Check sheet for the drawn part. Datum: minimum x, y, z corner. Units: mm. Round coordinates to 2 decimals unless told otherwise and drop trailing zeros. Write each loop counter-clockwise with the first axis right and the second up, starting at its lowest first coordinate (ties: lowest second). Pieces come first, ordered by that corner, then holes. Notation, with made-up numbers: M 65,35.5 L 83,35.5 A9 cw 83,48.5 Z; hole C -8,-4 d4. An arc over 180 degrees is marked long. One line per item, written item: value. Start each with the question number.
Item 1: Section check C-C, the plane y = 112. Record the cut outline in (x, z), then the cut area to 3 significant figures.
Item 2: Section check B-B, the plane z = 189. Record the cut outline in (x, y), then the cut area to 3 significant figures.
Item 3: Thickness scan on probe 1 along Z at (x, y) = (5.75, 103.5); probe 2 along Y at (x, z) = (1.5, 250); probe 3 along Y at (x, z) = (5.75, 187). Record the ranges inside material, lowest first. Write a range as from..to.
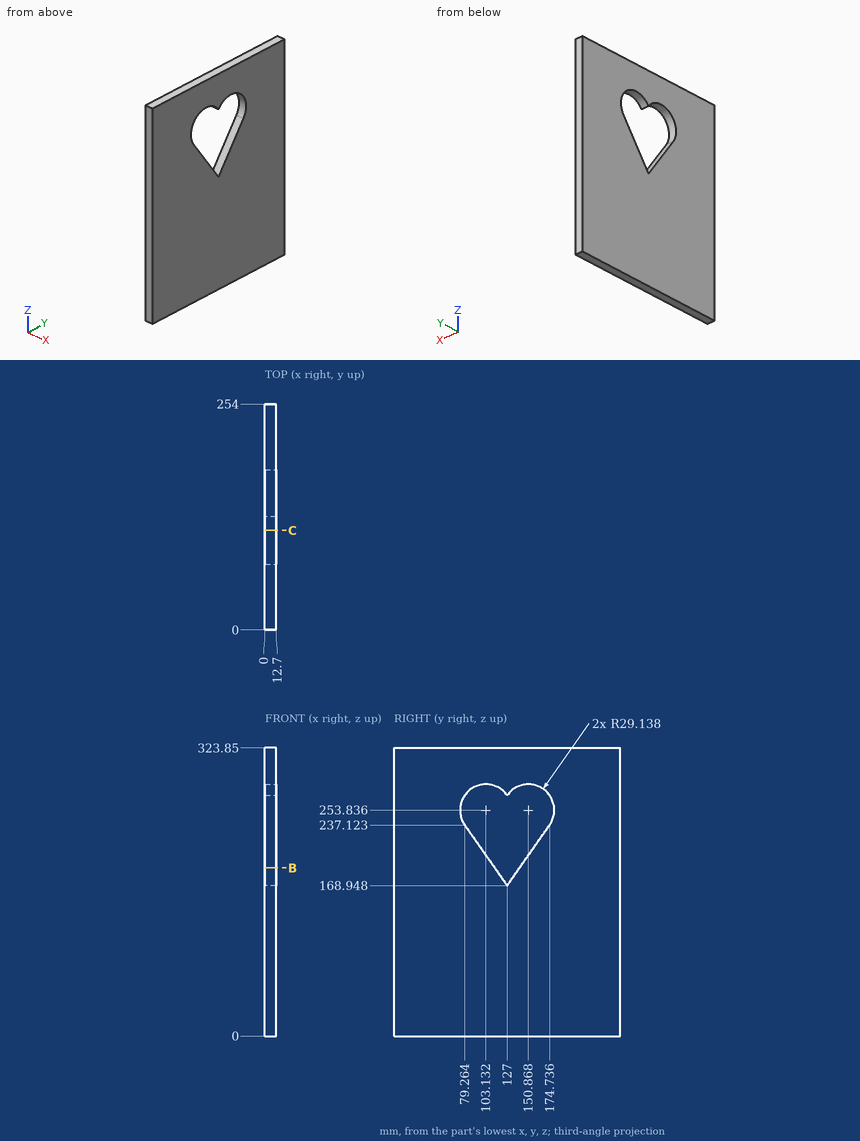
Response values:
1. outline: M 0,0 L 12.7,0 L 12.7,190.37 L 0,190.37 Z; M 0,281.59 L 12.7,281.59 L 12.7,323.85 L 0,323.85 Z
1. area: 2,950 mm2
2. outline: M 0,0 L 12.7,0 L 12.7,112.96 L 0,112.96 Z; M 0,141.04 L 12.7,141.04 L 12.7,254 L 0,254 Z
2. area: 2,870 mm2
3. probe 1: z = 0..202.51, 282.97..323.85
3. probe 2: y = 0..74.25, 179.75..254
3. probe 3: y = 0..114.36, 139.64..254
